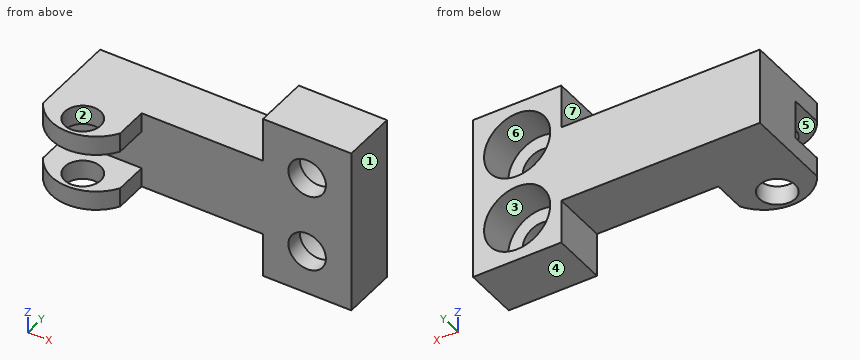
```python
from build123d import *

# Parameters (mm, degrees)
SKETCH_1_R                = 1.628497573
EXTRUDE_1_DEPTH           = 15
SKETCH_2_W                = 7
SKETCH_2_H                = 3.5
CUT_EXTRUDE_1_DEPTH       = 5
CUT_EXTRUDE_4_DEPTH       = 31.430248109
CUT_EXTRUDE_4_DEPTH_BACK  = 31.430248109
SKETCH_5_W                = 18
SKETCH_5_H                = 4
HOLE_WIZARD_1_D           = 3.4
HOLE_WIZARD_1_DEPTH       = 18.5
HOLE_WIZARD_1_CBORE_D     = 6
HOLE_WIZARD_1_CBORE_DEPTH = 3.4
HOLE_WIZARD_1_TIP         = 1.021463052


with BuildPart() as part:
    # 草图1 → 凸台-拉伸1 (new body)
    with BuildSketch(Plane.XY):
        with BuildLine():
            Line((0, 0), (-19, 0))
            Line((-19, 0), (-19, -3))
            ThreePointArc((-19, -3), (-22.5, -5), (-26, -3))
            Line((-26, -3), (-26, 0))
            Line((-26, 0), (-26, 5))
            Line((-26, 5), (0, 5))
            Line((0, 5), (0, 0))
        make_face()
        with Locations((-22.4, -3)):
            Circle(SKETCH_1_R, mode=Mode.SUBTRACT)
    extrude(amount=EXTRUDE_1_DEPTH)

    # 草图2 → 切除-拉伸1 (cut)
    with BuildSketch(Plane.XZ):
        with Locations((-22.5, 7.5)):
            Rectangle(SKETCH_2_W, SKETCH_2_H)
    extrude(amount=CUT_EXTRUDE_1_DEPTH, mode=Mode.SUBTRACT)

    # 草图5 → 切除-拉伸4 (cut, two sides: drawn at the far end of the back side and taken through both)
    with BuildSketch(Plane.XZ.offset(-CUT_EXTRUDE_4_DEPTH_BACK)):
        with Locations((-17, 13)):
            Rectangle(SKETCH_5_W, SKETCH_5_H)
        with Locations((-17, 2)):
            Rectangle(SKETCH_5_W, SKETCH_5_H)
    extrude(amount=CUT_EXTRUDE_4_DEPTH + CUT_EXTRUDE_4_DEPTH_BACK, mode=Mode.SUBTRACT)

    # 打孔尺寸(%根据)内六角圆柱头螺钉的类型1
    with Locations(Plane(origin=(-4, 5, 4), x_dir=(1, 0, 0), z_dir=(0, 1, 0))):
        with Locations((0, 0), (0, -7)):
            CounterBoreHole(HOLE_WIZARD_1_D / 2, HOLE_WIZARD_1_CBORE_D / 2, HOLE_WIZARD_1_CBORE_DEPTH, depth=HOLE_WIZARD_1_DEPTH)
            with Locations((0, 0, -(HOLE_WIZARD_1_DEPTH + HOLE_WIZARD_1_TIP / 2))):  # 118° drill point
                Cone(0, HOLE_WIZARD_1_D / 2, HOLE_WIZARD_1_TIP, mode=Mode.SUBTRACT)


solid = part.part
```
Input: part model. Units: mm. Frame: model coordinates. Face numbers are marked on the shaded views. A direction names the side the tool comes from. Give positions to 0.01 mm unless a question says otherwise; leave off trailing zeros. Loops run counter-clockwise (first coordinate to the right, second up) from the corner with the lowest first, then second, coordinate; pieces in that order, holes last. Notation, with made-up numbers: M 28.25,57 L 63.25,57 A28 ccw 63.25,77 Z; hole C 53.25,-11.75 d4. An arc over 180 degrees is marked long. Answer as CSV lines item,"result". Start each with the question number.
1. Pull-direction query (X, two-part tool) for the marked faces 1, 2, 3 and 4; classes: released by +X, released by -X, zero draft, split by the parting line, or undercut.
2. Section B-B on x = -4. Return loops of the section in (y, z).
3. Reachability of the marked faces 5, 6 and 7 from +Z, -Z, +X, -X, +Y, -Y: full face, straight path, thin tool, end or side. Return the list, or none.
4. Line query: L1, parallel to Z at x = -4, y = 0.4; L2, parallel to Z at x = -4, y = 3.55; L3, parallel to X at y = -3, z = 9.6. Output: solid intervals per line, ascending.
5. Section A-A on y = 2. Return loops of the section in (x, z).
6. Pin query (flat end, axial travel): P1, Ø3.5, axis at x = -4, z = 4, coming from the -Y side; P2, Ø4, axis at x = -24, y = -3, coming from the +Z side; P3, Ø2.5, axis at x = -22.4, y = -3, coming from the +Z side; P4, Ø5.5, axis at x = -21, y = -2.5, coming from the -Z side. Return the tip coordinate at first contact, or that it passes through.
7. Section D-D on y = -2. Return loops of the section in (x, z).
8. Section C-C on z = 4.5. Return loops of the section in (x, y) (1 decimal), plus the area to 3 significant figures.
Computed values:
1,face 1,"released by +X"
1,face 2,"undercut"
1,face 3,"undercut"
1,face 4,"zero draft"
2,outline,"M 0,0 L 5,0 L 5,1 L 1.6,1 L 1.6,2.3 L 0,2.3 Z; M 0,5.7 L 1.6,5.7 L 1.6,7 L 5,7 L 5,8 L 1.6,8 L 1.6,9.3 L 0,9.3 Z; M 0,12.7 L 1.6,12.7 L 1.6,14 L 5,14 L 5,15 L 0,15 Z"
3,face 5,"+X, -X, -Y"
3,face 6,"+Y"
3,face 7,"+Z, -X, +Y, -Y"
4,L1,"z = 0 to 2.3, 5.7 to 9.3, 12.7 to 15"
4,L2,"z = 0 to 1, 7 to 8, 14 to 15"
4,L3,"x = -26 to -24.03, -20.77 to -19"
5,outline,"M -26,4 L -8,4 L -8,0 L 0,0 L 0,15 L -8,15 L -8,11 L -26,11 Z; hole C -4,4 d6; hole C -4,11 d6"
6,P1,"stops at y = 0"
6,P2,"stops at z = 11"
6,P3,"passes through"
6,P4,"stops at z = 4"
7,outline,"M -26,4 L -23.69,4 L -23.69,5.75 L -26,5.75 Z; M -26,9.25 L -23.69,9.25 L -23.69,11 L -26,11 Z; M -21.11,4 L -19,4 L -19,5.75 L -21.11,5.75 Z; M -21.11,9.25 L -19,9.25 L -19,11 L -21.11,11 Z"
8,outline,"M -26,-3 A4.1 ccw -19,-3 L -19,0 L -5.6,0 L -5.6,1.6 L -7,1.6 L -7,5 L -26,5 Z; M -2.4,0 L 0,0 L 0,5 L -1,5 L -1,1.6 L -2.4,1.6 Z; hole C -22.4,-3 d3.3"
8,area,"127 mm²"
